```python
from build123d import *

# Parameters (mm, degrees)
F0_W     = 0.8
F0_H     = 5
F1_DEPTH = 13
F2_R     = 1
F3_DEPTH = 0.8
F4_SIZE  = 1


with BuildPart() as f1:
    # F0 (on Top) → F1 (new body)
    with BuildSketch(Plane.XY):
        with Locations((0.4, 2.5)):
            Rectangle(F0_W, F0_H)
    extrude(amount=F1_DEPTH)

    # F2 (on face) → F3 (cut, through all)
    with BuildSketch(Plane(origin=(0, 0, 0), x_dir=(0, -1, 0), z_dir=(-1, 0, 0))):
        with Locations((-2.5, 4)):
            Circle(F2_R)
    extrude(amount=-F3_DEPTH, mode=Mode.SUBTRACT)

    # F4
    f4_edges = [f1.edges().sort_by_distance(p)[0] for p in [
        (0.4, 5, 0),
        (0.4, 0, 0),
    ]]
    chamfer(f4_edges, length=F4_SIZE)


solid = f1.part
```
Model file for the job. Use its own axes, mm. Round coordinates to 2 decimals unless told otherwise and drop trailing zeros. Loops run counter-clockwise (first coordinate to the right, second up) from the corner with the lowest first, then second, coordinate; pieces in that order, holes last. Notation, with made-up numbers: M 67,-37.5 L 86,-37.5 A29 cw 86,-5.5 Z; hole C 79.25,-27 d11. An arc over 180 degrees is marked long. Put each result on its own line as item: value. Start each with the question number.
Item 1: Drop a flat-ended pin along its axis: P1, Ø1.6, axis at y = 2.5, z = 4, coming from the -X side. Give the stop position or say it passes through.
Item 2: Cut at C-C (x = 0.3). List the corners of the cut face in (y, z), then the cut area to 3 significant figures.
Item 3: Drill centre lines: line 1 along Z through (x, y) = (0.65, 2.5); line 2 along Z through (x, y) = (0.55, 2.9); line 3 along Z through (x, y) = (0.6, 0.95). Where is each one in solid material? Low to high.
Item 4: Mould opens along Y. For faces 1 (the face through (0.4, 0.5, 0.5)), 2 (the face through (0.4, 4.5, 0.5)), 3 (the face through (0.39, 2.63, 4.99)), 4 (the face through (0.8, 2, 6)) say: released by +Y, released by -Y, zero draft, split by the parting line, or undercut.
Item 5: Cut at B-B (y = 3.3). List the corners of the cut face in (x, z), then the cut area to 3 significant figures.
Item 6: Cut at D-D (y = 4.6). List the corners of the cut face in (x, z).
Item 7: Cut at A-A (z = 4). List the corners of the cut face in (x, y), then the cut area to 3 significant figures.
Answer block:
1. P1: through
2. outline: M 0,1 L 1,0 L 4,0 L 5,1 L 5,13 L 0,13 Z; hole C 2.5,4 d2
2. area: 60.9 mm2
3. line 1: 0 to 3, 5 to 13
3. line 2: 0 to 3.08, 4.92 to 13
3. line 3: 0.05 to 13
4. face 1: released by -Y
4. face 2: released by +Y
4. face 3: undercut
4. face 4: zero draft
5. outline: M 0,0 L 0.8,0 L 0.8,3.4 L 0,3.4 Z; M 0,4.6 L 0.8,4.6 L 0.8,13 L 0,13 Z
5. area: 9.44 mm2
6. outline: M 0,0.6 L 0.8,0.6 L 0.8,13 L 0,13 Z
7. outline: M 0,0 L 0.8,0 L 0.8,1.5 L 0,1.5 Z; M 0,3.5 L 0.8,3.5 L 0.8,5 L 0,5 Z
7. area: 2.40 mm2
